from build123d import *

# Parameters (mm, degrees)
F0_W     = 60
F0_H     = 100
F1_DEPTH = 100
F2_R     = 6
F3_DEPTH = 100
F4_R     = 6
F5_DEPTH = 65
F6_W     = 25
F6_H     = 17.1061154245
F7_ANGLE = 180


with BuildPart() as f1:
    # F0 (on Top) → F1 (new body)
    with BuildSketch(Plane.XY):
        Rectangle(F0_W, F0_H)
    extrude(amount=F1_DEPTH)

    # F2 (on face) → F3 (cut)
    with BuildSketch(Plane.XY.offset(100)):
        with Locations((0, 35)):
            Circle(F2_R)
        with Locations((0, -35)):
            Circle(F2_R)
    extrude(amount=-F3_DEPTH, mode=Mode.SUBTRACT)

    # F4 (on face) → F5 (cut)
    with BuildSketch(Plane.XY.offset(100)):
        Polygon((-30, 50), (-30, 17.8938845755), (-5, 17.8938845755), (-5, -17.1061154245), (-30, -17.1061154245), (-30, -50), (30, -50), (30, 50), align=None)
        with Locations((0, -35)):
            Circle(F4_R, mode=Mode.SUBTRACT)
        with Locations((0, 35)):
            Circle(F4_R, mode=Mode.SUBTRACT)
    extrude(amount=-F5_DEPTH, mode=Mode.SUBTRACT)

    # F6 (on face) → F7 (revolve)
    with BuildSketch(Plane.XY.offset(100)):
        with Locations((-17.5, -8.5530577123)):
            Rectangle(F6_W, F6_H)
    revolve(axis=Axis((-17.5, 0, 100), (-1, 0, 0)), revolution_arc=F7_ANGLE)


solid = f1.part
Build history of the part. All positions in model axes, mm. A direction names the side the tool comes from. Give positions to 0.01 mm unless a question says otherwise; leave off trailing zeros. Loops run counter-clockwise (first coordinate to the right, second up) from the corner with the lowest first, then second, coordinate; pieces in that order, holes last. Notation, with made-up numbers: (17, 49.25) - (57, 49.25) arc R24 cw to (57, 80.25) - close; hole circle Ø1 at (-23.75, 80). An arc over 180 degrees is marked (long way). Write item = value, one per line. Start each with the question number.
1) Band-saw the part on C-C on x = 1. Give the cut face in (y, z), plus the area to 3 significant figures.
2) Probe probe 1 along Y at (x, z) = (0, 14.5); probe 2 along Y at (x, z) = (-2, 7); probe 3 along Z at (x, y) = (6.5, 25.5). List the from-to ranges inside material, lowest first. Write a range as from..to.
3) Pull direction X, two halves, no side cores. Call faces 4 (the flat face through (-5, 1, 77)), 5 (the flat face through (-30, 1, 46)), 6 (the flat face through (0, 1, 0)), 7 (the cylindrical face through (-1.301, 29.143, 17.745)): +X half, -X half, draft (parallel to the pull), parting line (faces both ways), or undercut.
4) Drop flat-ended pins along their axis: pin 1 Ø12.5 at (x, z) = (-14, 56) entering from -Y; pin 2 Ø9.5 at (x, y) = (0, -35) entering from -Z; pin 3 Ø4 at (x, y) = (-11.5, 37) entering from +Z; pin 4 Ø5 at (x, y) = (19.5, 1.5) entering from -Z. Give the stop position or say it passes through.
5) Band-saw the part on A-A on y = -35. Give the cut face in (x, z).
6) Band-saw the part on B-B on x = -19. Give the cut face in (y, z).
7) Band-saw the part on D-D on y = 0. Give the cut face in (x, z).
8) Tool access for faces 1 (the flat face through (-18, 17.894, 68)), 2 (the flat face through (0, -50, 17)), 3 (the flat face through (-17, -17.106, 68)): list every direction of +Z, -Z, +X, -X, +Y, -Y with a clear straight run to the whole face (end or side of a thin tool).
Final values:
q1.outline = (-50, 0) - (-40.92, 0) - (-40.92, 35) - (-50, 35) - close; (-29.08, 0) - (29.08, 0) - (29.08, 35) - (-29.08, 35) - close; (40.92, 0) - (50, 0) - (50, 35) - (40.92, 35) - close
q1.area = 2,670 mm²
q2.probe_1 = -50..-41, -29..29, 41..50
q2.probe_2 = -50..-40.66, -29.34..29.34, 40.66..50
q2.probe_3 = 0..35
q3.face_4 = +X half
q3.face_5 = -X half
q3.face_6 = draft
q3.face_7 = undercut
q4.pin_1 = -17.11
q4.pin_2 = through
q4.pin_3 = 35
q4.pin_4 = 0
q5.outline = (-30, 0) - (-6, 0) - (-6, 35) - (-30, 35) - close; (6, 0) - (30, 0) - (30, 35) - (6, 35) - close
q6.outline = (-50, 0) - (50, 0) - (50, 35) - (17.89, 35) - (17.89, 100) - (17.11, 100) arc R17.11 ccw to (-17.11, 100) - (-17.11, 35) - (-50, 35) - close
q7.outline = (-30, 0) - (30, 0) - (30, 35) - (-5, 35) - (-5, 117.11) - (-30, 117.11) - close
q8.face_1 = +Z, +X, -X, +Y
q8.face_2 = +Z, -Z, +X, -X, -Y
q8.face_3 = +Z, +X, -X, -Y
